Autodesk Inventor part; units mm, degrees
ref_plane "YZ Plane" through (0, 0, 0) normal (1, 0, 0) x (0, 1, 0)
ref_plane "XZ Plane" through (0, 0, 0) normal (0, 1, 0) x (-1, 0, 0)
ref_plane "XY Plane" through (0, 0, 0) normal (0, 0, 1) x (1, 0, 0)
sketch "Sketch1" plane through (0, 0, 0) normal (1, 0, 0) x (0, 1, 0)
  line L0 (0.019, 0.9702) -> (3.175, 0.9702)
  line L1 (3.175, 0.9702) -> (3.175, -2.3953)
  line L2 (0.019, 9.2838) -> (0.019, -29.9451)
  line L3 (3.175, -2.3953) -> (0.019, -2.3953)
  point P0 (0, 0)
  dimension "d3" = 3.1559
  dimension "d4" = 3.3655
revolve "Revolution1" add sketch "Sketch1" angle 360 about axis through (0, 0.019, 9.2838) along (0, 0, -1)
sketch "Sketch3" plane through (0, 0.019, 0.9702) normal (0, 0, 1) x (1, 0, 0)
  circle A0 centre (0, 0) radius 5.715
  point P0 (0, -0.019)
extrude "Extrusion2" add sketch "Sketch3" along normal blind 0.635
sketch "Sketch4" plane through (0, 0.019, 1.6052) normal (0, 0, 1) x (1, 0, 0)
  point P0 (0, -0.019)
  point P1 (0, -0.019)
hole "Hole2" at (0, 0, 1.6052) direction (0, 0, -1) diameter 3.556 end through all
properties part number "bearing"
Input: part model. Units: mm. Frame: model coordinates. A direction names the side the tool comes from. Coordinates: 2 decimals unless noted, no trailing zeros. Write each loop counter-clockwise with the first axis right and the second up, starting at its lowest first coordinate (ties: lowest second). Pieces come first, ordered by that corner, then holes.
1) Mould query, pull axis Y, two halves, no side actions, for faces 1 (the flat face through (2.5, -2.4, 0.97)), 2 (the cylindrical face through (1.736, 0.385, -0.423)), 3 (the cylindrical face through (-1.239, 5.598, 1.283)). Classes: pulls with the +Y half, pulls with the -Y half, needs draft (parallel to the pull), parting line crosses it, or undercut.
2) Section C-C on y = 2.25. Output: boundary loops of the cut face in (x, z), and give its area (3 significant figures).
3) Material intervals for line 1 along X through (y, z) = (0, -0.95); line 2 along Z through (x, y) = (-1, 4.25); line 3 along X through (y, z) = (-1.25, -2.15), sorted ascending.
4) Pin query (flat end, axial travel): pin 1 Ø1 at (x, z) = (-4, 1) entering from -Y; pin 2 Ø2 at (x, z) = (-3.5, 0.5) entering from -Y. Return the tip coordinate at first contact, or that it passes through.
5) Section D-D on x = -1.5. Output: boundary loops of the cut face in (y, z).
6) Set-up query: faces 4 (the flat face through (-1.4, 1.4, 1.605)), 5 (the cylindrical face through (-3.08, -0.67, -0.74)). Return all of +Z, -Z, +X, -X, +Y, -Y with unobstructed straight access to the full face (end or side cutting, diameter ignored); none if empty.
7) Section B-B on z = 0.35. Output: boundary loops of the cut face in (x, y) (3 decimals).
8) Section A-A on x = 0. Output: boundary loops of the cut face in (y, z) (3 decimals).
Check result:
1. face 1: needs draft
1. face 2: undercut
1. face 3: parting line crosses it
2. outline: (-5.26, 0.97) - (-2.23, 0.97) - (-2.23, -2.4) - (2.23, -2.4) - (2.23, 0.97) - (5.26, 0.97) - (5.26, 1.61) - (-5.26, 1.61) - close
2. area: 21.7 mm2
3. line 1: x = -3.16 to -1.78, 1.78 to 3.16
3. line 2: z = 0.97 to 1.61
3. line 3: x = -2.89 to -1.26, 1.26 to 2.89
4. pin 1: stops at y = -4.5
4. pin 2: stops at y = -5.06
5. outline: (-5.5, 0.97) - (-2.76, 0.97) - (-2.76, -2.4) - (-0.95, -2.4) - (-0.95, 1.61) - (-5.5, 1.61) - close; (0.95, -2.4) - (2.8, -2.4) - (2.8, 0.97) - (5.53, 0.97) - (5.53, 1.61) - (0.95, 1.61) - close
6. face 4: +Z, +X, -X, +Y, -Y
6. face 5: -Z
7. outline: circle Ø6.312 at (0, 0.019); hole circle Ø3.556 at (0, 0)
8. outline: (-5.696, 0.97) - (-3.137, 0.97) - (-3.137, -2.395) - (-1.778, -2.395) - (-1.778, 1.605) - (-5.696, 1.605) - close; (1.778, -2.395) - (3.175, -2.395) - (3.175, 0.97) - (5.734, 0.97) - (5.734, 1.605) - (1.778, 1.605) - close
